Geometry: final body of the model. Coordinates: model frame, mm. A direction names the side the tool comes from. Coordinates: 2 decimals unless noted, no trailing zeros. Write each loop counter-clockwise with the first axis right and the second up, starting at its lowest first coordinate (ties: lowest second). Pieces come first, ordered by that corner, then holes. Notation, with made-up numbers: M -26,-6.75 L 0,-6.75 A15 ccw 0,16.25 Z; hole C 87,-23.5 d10. An arc over 180 degrees is marked long. Write item = value, one per line. Start each with the question number.
Item 1: Section A-A on x = 13.5. Output: boundary loops of the cut face in (y, z).
Item 2: Section B-B on y = 6. Output: boundary loops of the cut face in (x, z), plus the area to 3 significant figures.
Item 3: Section C-C on z = 3. Output: boundary loops of the cut face in (x, y), plus the area to 3 significant figures.
Item 4: First-contact query: pin 1 Ø8 at (x, y) = (55, 6) entering from +Z; pin 2 Ø7.5 at (y, z) = (7.5, 3.5) entering from +X. Flat tips, straight axial feed; report the tip coordinate or a pass-through.
Item 5: Reachability of faces 1 (the cylindrical face through (4, 18.4, 2.4)), 2 (the cylindrical face through (0.57, 8.62, -33.4)), 3 (the flat face through (36, 8, 0)) from +Z, -Z, +X, -X, +Y, -Y: full face, straight path, thin tool, end or side. Return the list, or none.
Item 6: Ray query, L1, parallel to X at y = 9.5, z = 0.5; L2, parallel to Z at x = 39, y = 12.25; L3, parallel to X at y = 17.5, z = -10. Return the intervals inside material, ascending. Write a range as [from, to].
from build123d import *

# Parameters (mm, degrees)
SKETCH1_W           = 70
SKETCH1_H           = 34
BOSS_EXTRUDE1_DEPTH = 19
SKETCH2_W           = 4.574362022
SKETCH2_H           = 19
BOSS_EXTRUDE2_DEPTH = 7
FILLET2_R           = 2
FILLET3_R           = 2


with BuildPart() as part:
    # Sketch1 → Boss-Extrude1 (new body)
    with BuildSketch(Plane(origin=(0, 0, 0), x_dir=(1, 0, 0), z_dir=(0, 1, 0))):
        with Locations((35, 17)):
            Rectangle(SKETCH1_W, SKETCH1_H)
    extrude(amount=BOSS_EXTRUDE1_DEPTH)

    # Sketch2 → Boss-Extrude2 (add)
    with BuildSketch(Plane.XY):
        with Locations((2.287181011, 9.5)):
            Rectangle(SKETCH2_W, SKETCH2_H)
    extrude(amount=BOSS_EXTRUDE2_DEPTH)

    # Fillet2
    fillet2_edges = [part.edges().sort_by_distance(p)[0] for p in [
        (35, 19, -34),
        (37.287181011, 19, 0),
    ]]
    fillet(fillet2_edges, radius=FILLET2_R)

    # Fillet3
    fillet3_edges = [part.edges().sort_by_distance(p)[0] for p in [
        (0, 8.5, -34),
        (0, 18.414213562, -33.414213562),
        (70, 8.5, 0),
        (70, 18.414213562, -0.585786438),
        (70, 18.414213562, -33.414213562),
        (4.574362022, 19, 2.5),
        (2.287181011, 19, 7),
        (0, 19, -12.5),
        (70, 19, -17),
        (70, 8.5, -34),
    ]]
    fillet(fillet3_edges, radius=FILLET3_R)


solid = part.part
Responses:
q1.outline = M 0,-34 L 17,-34 A2 ccw 19,-32 L 19,-2 A2 ccw 17,0 L 0,0 Z
q2.outline = M 0,-32 A2 ccw 2,-34 L 68,-34 A2 ccw 70,-32 L 70,-2 A2 ccw 68,0 L 4.57,0 L 4.57,7 L 0,7 Z
q2.area = 2,410 mm²
q3.outline = M 0,0 L 4.57,0 L 4.57,17 A2 ccw 2.57,19 L 2,19 A2 ccw 0,17 Z
q3.area = 85.2 mm²
q4.pin_1 = 0
q4.pin_2 = 68.97
q5.face_1 = +Z, +X, +Y
q5.face_2 = -Z, -X, +Y, -Y
q5.face_3 = +Z, +X, +Y, -Y
q6.L1 = [0, 4.57]
q6.L2 = [-34, 0]
q6.L3 = [0.06, 69.94]
